CAD build for the part. Positions are in the model's coordinates, mm. A direction names the side the tool comes from. Give positions to 0.01 mm unless a question says otherwise; leave off trailing zeros. Loops run counter-clockwise (first coordinate to the right, second up) from the corner with the lowest first, then second, coordinate; pieces in that order, holes last.
Item 1: Which spindle directions (+Z, -Z, +X, -X, +Y, -Y) get a long thin tool onto all of the face, cutting with end or side? Do faces 4 (the flat face through (-57, -1.25, 0)), 5 (the cylindrical face through (51.45, -0.49, -10.07)), 6 (the cylindrical face through (50.661, -1.76, -12.097)). Say none if no direction does.
Item 2: Saw through at A-A on x = 53.2. Give the cut face in (y, z), plus the area to 4 significant figures.
Item 3: Saw through at C-C on z = -10.15. Give the cut face in (x, y).
Item 4: Saw through at B-B on y = -1.8. Give the cut face in (x, z), plus the area to 3 significant figures.
Item 5: Mould opens along Z. For faces 1 (the flat face through (-52, -1, -12)), 2 (the cylindrical face through (-57.4, -1.23, 17.89)), 3 (the flat face through (58.3, -1, 0)) say: released by +Z, released by -Z, zero draft, split by the parting line, or undercut.
Item 6: Probe probe 1 along Z at (x, y) = (53.2, -0.75); probe 2 along Z at (x, y) = (53.2, -1.45); probe 3 along X at (y, z) = (-0.7, 10.15). List the from-to ranges inside material, lowest first.
Item 7: Drop flat-ended pins along their axis: P1, Ø1.9, axis at x = -52.5, z = -11, coming from the -Y side; P2, Ø3, axis at x = 53.2, z = 10.15, coming from the +Y side; P3, Ø0.6, axis at x = -57.5, y = -0.5, coming from the +Z side. Give the stop position or say it passes through.
from build123d import *

# Parameters (mm, degrees)
F0_R     = 1.75
F1_DEPTH = 2.5
F2_R     = 3.2
F3_DEPTH = 1.5
F4_W     = 2.5
F4_H     = 6
F5_DEPTH = 1.25


with BuildPart() as f1:
    # F0 (on Front) → F1 (new body)
    with BuildSketch(Plane.XZ):
        with BuildLine():
            Line((55.3, 18.75), (-55.3, 18.75))
            ThreePointArc((-55.3, 18.75), (-57.42132, 17.87132), (-58.3, 15.75))
            Line((-58.3, 15.75), (-58.3, -15.75))
            ThreePointArc((-58.3, -15.75), (-57.42132, -17.87132), (-55.3, -18.75))
            Line((-55.3, -18.75), (55.3, -18.75))
            ThreePointArc((55.3, -18.75), (57.42132, -17.87132), (58.3, -15.75))
            Line((58.3, -15.75), (58.3, 15.75))
            ThreePointArc((58.3, 15.75), (57.42132, 17.87132), (55.3, 18.75))
        make_face()
        with Locations((-53.2, -10.15)):
            Circle(F0_R, mode=Mode.SUBTRACT)
        with Locations((53.2, -10.15)):
            Circle(F0_R, mode=Mode.SUBTRACT)
        with Locations((-53.2, 10.15)):
            Circle(F0_R, mode=Mode.SUBTRACT)
        with Locations((53.2, 10.15)):
            Circle(F0_R, mode=Mode.SUBTRACT)
    extrude(amount=F1_DEPTH)

    # F2 (on face) → F3 (cut)
    with BuildSketch(Plane.XZ.offset(2.5)):
        with Locations((-53.2, 10.15)):
            Circle(F2_R)
        with Locations((53.2, 10.15)):
            Circle(F2_R)
        with Locations((-53.2, -10.15)):
            Circle(F2_R)
        with Locations((53.2, -10.15)):
            Circle(F2_R)
    extrude(amount=-F3_DEPTH, mode=Mode.SUBTRACT)

    # F4 (on face) → F5 (cut)
    with BuildSketch(Plane(origin=(0, 0, 0), x_dir=(-1, 0, 0), z_dir=(0, 1, 0))):
        with Locations((57.05, 0)):
            Rectangle(F4_W, F4_H)
    extrude(amount=-F5_DEPTH, mode=Mode.SUBTRACT)


solid = f1.part
Results below:
1. face 4: -X, +Y
1. face 5: +Y, -Y
1. face 6: -Y
2. outline: (-2.5, -18.75) - (0, -18.75) - (0, -11.9) - (-1, -11.9) - (-1, -13.35) - (-2.5, -13.35) - close; (-2.5, -6.95) - (-1, -6.95) - (-1, -8.4) - (0, -8.4) - (0, 8.4) - (-1, 8.4) - (-1, 6.95) - (-2.5, 6.95) - close; (-2.5, 13.35) - (-1, 13.35) - (-1, 11.9) - (0, 11.9) - (0, 18.75) - (-2.5, 18.75) - close
2. area: 67.55 mm2
3. outline: (-58.3, -2.5) - (-56.4, -2.5) - (-56.4, -1) - (-54.95, -1) - (-54.95, 0) - (-58.3, 0) - close; (-51.45, -1) - (-50, -1) - (-50, -2.5) - (50, -2.5) - (50, -1) - (51.45, -1) - (51.45, 0) - (-51.45, 0) - close; (54.95, -1) - (56.4, -1) - (56.4, -2.5) - (58.3, -2.5) - (58.3, 0) - (54.95, 0) - close
4. outline: (-58.3, -15.75) arc R3 ccw to (-55.3, -18.75) - (55.3, -18.75) arc R3 ccw to (58.3, -15.75) - (58.3, 15.75) arc R3 ccw to (55.3, 18.75) - (-55.3, 18.75) arc R3 ccw to (-58.3, 15.75) - close; hole circle Ø6.4 at (-53.2, -10.15); hole circle Ø6.4 at (-53.2, 10.15); hole circle Ø6.4 at (53.2, -10.15); hole circle Ø6.4 at (53.2, 10.15)
4. area: 4,240 mm2
5. face 1: undercut
5. face 2: released by +Z
5. face 3: zero draft
6. probe 1: z = -18.75 to -11.9, -8.4 to 8.4, 11.9 to 18.75
6. probe 2: z = -18.75 to -13.35, -6.95 to 6.95, 13.35 to 18.75
6. probe 3: x = -58.3 to -54.95, -51.45 to 51.45, 54.95 to 58.3
7. P1: stops at y = -1
7. P2: passes through
7. P3: stops at z = 18.07
